```python
from build123d import *

# Parameters (mm, degrees)
BOSS_EXTRUDE1_DEPTH      = 15
BOSS_EXTRUDE1_DEPTH_BACK = 15
SKETCH2_R                = 3
CUT_EXTRUDE1_DEPTH       = 83.324054808
FILLET1_R                = 5
CUT_EXTRUDE2_START       = -28.5
SKETCH3_W                = 5
SKETCH3_H                = 18
CUT_EXTRUDE2_DEPTH       = 28.5
CUT_EXTRUDE3_DEPTH       = 83.324054808
CUT_EXTRUDE3_DEPTH_BACK  = 83.324054808
SKETCH4_R                = 3
SKETCH5_R                = 2
CUT_EXTRUDE4_DEPTH       = 83.324054808


with BuildPart() as part:
    # Sketch1 → Boss-Extrude1 (new, two sides: drawn at the far end of the back side and taken through both)
    with BuildSketch(Plane.XY.offset(-BOSS_EXTRUDE1_DEPTH_BACK)):
        Polygon((-72.5, 34), (-72.5, 0), (72.5, 0), (72.5, 36), (56.5, 36), (56.5, 6), (-66, 6), (-66, 34), align=None)
    extrude(amount=BOSS_EXTRUDE1_DEPTH + BOSS_EXTRUDE1_DEPTH_BACK)

    # Sketch2 → Cut-Extrude1 (cut, through all)
    with BuildSketch(Plane(origin=(0, 0, 0), x_dir=(1, 0, 0), z_dir=(0, 1, 0))):
        with Locations(Location((-57.5, 0, 0), (0, 0, 180))):
            Circle(SKETCH2_R)
        with Locations(Location((64.5, 0, 0), (0, 0, 270))):
            Circle(SKETCH2_R)
    extrude(amount=CUT_EXTRUDE1_DEPTH, mode=Mode.SUBTRACT)

    # Fillet1
    fillet1_edges = [part.edges().sort_by_distance(p)[0] for p in [
        (-66, 6, 0),
        (56.5, 6, 0),
    ]]
    fillet(fillet1_edges, radius=FILLET1_R)

    # Sketch3 → Cut-Extrude2 (cut)
    with BuildSketch(Plane(origin=(0, 36, 0), x_dir=(1, 0, 0), z_dir=(0, 1, 0)).offset(CUT_EXTRUDE2_START)):
        with BuildLine():
            Line((72.5, 9), (56.5, 9))
            Line((56.5, 9), (56.5, -9))
            Line((56.5, -9), (62.506908484, -2.242227956))
            ThreePointArc((62.506908484, -2.242227956), (62.257772044, 1.993091516), (66.493091516, 2.242227956))
            Line((66.493091516, 2.242227956), (72.5, 9))
        make_face()
        with Locations((54, 0)):
            Rectangle(SKETCH3_W, SKETCH3_H)
        with BuildLine():
            Line((72.5, -9), (72.5, 9))
            Line((72.5, 9), (66.493091516, 2.242227956))
            ThreePointArc((66.493091516, 2.242227956), (67.236720167, 1.228968155), (67.5, 0))
            ThreePointArc((67.5, 0), (65.728968155, -2.736720167), (62.506908484, -2.242227956))
            Line((62.506908484, -2.242227956), (56.5, -9))
            Line((56.5, -9), (72.5, -9))
        make_face()
    extrude(amount=CUT_EXTRUDE2_DEPTH, mode=Mode.SUBTRACT)

    # Sketch4 → Cut-Extrude3 (cut, two sides: drawn at the far end of the back side and taken through both)
    with BuildSketch(Plane.XY.offset(-CUT_EXTRUDE3_DEPTH_BACK)):
        with Locations((65.25, 26.25)):
            Circle(SKETCH4_R)
    extrude(amount=CUT_EXTRUDE3_DEPTH + CUT_EXTRUDE3_DEPTH_BACK, mode=Mode.SUBTRACT)

    # Sketch5 → Cut-Extrude4 (cut, through all)
    with BuildSketch(Plane(origin=(0, 0, 0), x_dir=(0, 0, -1), z_dir=(1, 0, 0))):
        with Locations((0, 27)):
            Circle(SKETCH5_R)
    extrude(amount=-CUT_EXTRUDE4_DEPTH, mode=Mode.SUBTRACT)


solid = part.part
```
Part model, mm, in its own coordinate system. A direction names the side the tool comes from. Round coordinates to 2 decimals unless told otherwise and drop trailing zeros. Loops run counter-clockwise (first coordinate to the right, second up) from the corner with the lowest first, then second, coordinate; pieces in that order, holes last.
Item 1: 3-axis set-ups, long thin cutter, end or side, ignore diameter. For faces 1 (the face through (-69, 34, 0)), 2 (the face through (64, 22, -9)), 3 (the face through (54.413, 6.936, 0.21)), 4 (the face through (65, 36, -12)): which of +Z, -Z, +X, -X, +Y, -Y reach the whole face in a straight line?
Item 2: Mould opens along X. For faces 5 (the face through (64, 22, 9)), 6 (the face through (-72.5, 17, 0)), 7 (the face through (56.5, 24, -12)), 8 (the face through (72.5, 6, 0)) say: +X half, -X half, draft (parallel to the pull), parting line (faces both ways), or undercut.
Item 3: Cut at B-B, the plane x = -57.5. Give the cut face in (y, z), then the cut area to 3 significant figures.
Item 4: Drop flat-ended pins along their axis: P1, Ø7, axis at x = 65.25, y = 26.25, coming from the +Z side; P2, Ø15, axis at x = 2, z = -3.5, coming from the +Y side; P3, Ø2.5, axis at y = 27, z = 0, coming from the +X side; P4, Ø5, axis at x = 61, z = -3, coming from the +Y side. Give the stop position or say it passes through.
Item 5: Cut at A-A, the plane z = 0. Give the cut face in (x, y).
Item 6: Cut at C-C, the plane y = 20.5. Give the cut face in (x, z), then the cut area to 3 significant figures.
Item 7: Cut at D-D, the plane z = -11.25. Give the cut face in (x, y), then the cut area to 3 significant figures.
Item 8: Drill centre lines: line 1 (X direction, y = 2.3, z = 0); line 2 (X direction, y = 26.25, z = 12.8); line 3 (Y direction, x = 65.25, z = -11.6). Where is each one in solid material? Low to high.
A:
1. face 1: +Z, -Z, -X, +Y
1. face 2: +X, +Y
1. face 3: +Z, -Z, +Y
1. face 4: +Z, -Z, +X, -X, +Y
2. face 5: draft
2. face 6: -X half
2. face 7: undercut
2. face 8: +X half
3. outline: (0, -15) - (6, -15) - (6, -3) - (0, -3) - close; (0, 3) - (6, 3) - (6, 15) - (0, 15) - close
3. area: 144 mm2
4. P1: stops at z = 15
4. P2: stops at y = 6
4. P3: passes through
4. P4: stops at y = 7.5
5. outline: (-72.5, 0) - (-60.5, 0) - (-60.5, 6) - (-61, 6) arc R5 cw to (-66, 11) - (-66, 25) - (-72.5, 25) - close; (-72.5, 29) - (-66, 29) - (-66, 34) - (-72.5, 34) - close; (-54.5, 0) - (61.5, 0) - (61.5, 7.5) - (55.07, 7.5) arc R5 cw to (51.5, 6) - (-54.5, 6) - close; (67.5, 0) - (72.5, 0) - (72.5, 7.5) - (67.5, 7.5) - close
6. outline: (-72.5, -15) - (-66, -15) - (-66, 15) - (-72.5, 15) - close; (56.5, -15) - (72.5, -15) - (72.5, -9) - (56.5, -9) - close; (56.5, 9) - (72.5, 9) - (72.5, 15) - (56.5, 15) - close
6. area: 387 mm2
7. outline: (-72.5, 0) - (72.5, 0) - (72.5, 36) - (56.5, 36) - (56.5, 11) arc R5 cw to (51.5, 6) - (-61, 6) arc R5 cw to (-66, 11) - (-66, 34) - (-72.5, 34) - close; hole circle Ø6 at (65.25, 26.25)
7. area: 1,510 mm2
8. line 1: x = -72.5 to -60.5, -54.5 to 61.5, 67.5 to 72.5
8. line 2: x = -72.5 to -66, 56.5 to 62.25, 68.25 to 72.5
8. line 3: y = 0 to 23.25, 29.25 to 36
